Could you check a few things on this model? Use its own coordinates, in mm. A direction names the side the tool comes from. Give positions to 0.01 mm unless a question says otherwise; leave off trailing zeros. Order: outer loops, then holes, each group sorted by start corner. A loop starts at its lowest first (then second) coordinate and runs counter-clockwise, first axis right, second up. Notation, with made-up numbers: (18, 28) -> (61, 28) arc R16 cw to (61, 33) -> close; hole circle Ø1 at (38, -30). An arc over 180 degrees is marked (long way). One line per item, written item: value.
```python
from build123d import *

# Parameters (mm, degrees)
SKETCH1_R           = 1.75
BOSS_EXTRUDE1_DEPTH = 2


with BuildPart() as part:
    # Sketch1 → Boss-Extrude1 (new body)
    with BuildSketch(Plane(origin=(0, 0, 0), x_dir=(1, 0, 0), z_dir=(0, 1, 0))):
        with BuildLine():
            Line((-12.5, -149.799866489), (-12.5, -72.328332691))
            ThreePointArc((-12.5, -72.328332691), (-11.914213562, -70.914119129), (-10.5, -70.328332691))
            Line((-10.5, -70.328332691), (10.5, -70.328332691))
            ThreePointArc((10.5, -70.328332691), (11.914213562, -70.914119129), (12.5, -72.328332691))
            Line((12.5, -72.328332691), (12.5, -149.799866489))
            ThreePointArc((12.5, -149.799866489), (13.155638081, -151.280640283), (14.69269103, -151.790562389))
            ThreePointArc((14.69269103, -151.790562389), (132.068874077, -76.25), (138.800828598, 63.171037513))
            ThreePointArc((138.800828598, 63.171037513), (137.590696626, 64.247203361), (135.980489863, 64.074615697))
            Line((135.980489863, 64.074615697), (68.888173524, 25.338848798))
            ThreePointArc((68.888173524, 25.338848798), (67.370535433, 25.139047953), (66.156122716, 26.070899606))
            Line((66.156122716, 26.070899606), (55.656122716, 44.257433085))
            ThreePointArc((55.656122716, 44.257433085), (55.456321871, 45.775071175), (56.388173524, 46.989483893))
            Line((56.388173524, 46.989483893), (123.480489863, 85.725250792))
            ThreePointArc((123.480489863, 85.725250792), (124.435058545, 87.033436922), (124.108137568, 88.619524876))
            ThreePointArc((124.108137568, 88.619524876), (0, 152.5), (-124.108137568, 88.619524876))
            ThreePointArc((-124.108137568, 88.619524876), (-124.435058545, 87.033436922), (-123.480489863, 85.725250792))
            Line((-123.480489863, 85.725250792), (-56.388173524, 46.989483893))
            ThreePointArc((-56.388173524, 46.989483893), (-55.456321871, 45.775071175), (-55.656122716, 44.257433085))
            Line((-55.656122716, 44.257433085), (-66.156122716, 26.070899606))
            ThreePointArc((-66.156122716, 26.070899606), (-67.370535433, 25.139047953), (-68.888173524, 25.338848798))
            Line((-68.888173524, 25.338848798), (-135.980489863, 64.074615697))
            ThreePointArc((-135.980489863, 64.074615697), (-137.590696626, 64.247203361), (-138.800828598, 63.171037513))
            ThreePointArc((-138.800828598, 63.171037513), (-132.068874077, -76.25), (-14.69269103, -151.790562389))
            ThreePointArc((-14.69269103, -151.790562389), (-13.155638081, -151.280640283), (-12.5, -149.799866489))
        make_face()
        with Locations(Location((115.282765815, -66.558535876, 0), (0, 0, 270))):
            Circle(SKETCH1_R, mode=Mode.SUBTRACT)
        with Locations(Location((102.292384759, -59.058535876, 0), (0, 0, 270))):
            Circle(SKETCH1_R, mode=Mode.SUBTRACT)
        with Locations(Location((-115.282765815, -66.558535876, 0), (0, 0, 270))):
            Circle(SKETCH1_R, mode=Mode.SUBTRACT)
        with Locations(Location((-102.292384759, -59.058535876, 0), (0, 0, 270))):
            Circle(SKETCH1_R, mode=Mode.SUBTRACT)
        with Locations(Location((0, 133.117071753, 0), (0, 0, 270))):
            Circle(SKETCH1_R, mode=Mode.SUBTRACT)
        with Locations(Location((0, 118.117071753, 0), (0, 0, 270))):
            Circle(SKETCH1_R, mode=Mode.SUBTRACT)
        with Locations(Location((110.01987893, 90.400875942, 0), (0, 0, 270))):
            Circle(SKETCH1_R, mode=Mode.SUBTRACT)
        with Locations(Location((85.771167624, 76.400875942, 0), (0, 0, 270))):
            Circle(SKETCH1_R, mode=Mode.SUBTRACT)
        with Locations(Location((133.29987893, 50.078733142, 0), (0, 0, 270))):
            Circle(SKETCH1_R, mode=Mode.SUBTRACT)
        with Locations(Location((109.051167624, 36.078733142, 0), (0, 0, 270))):
            Circle(SKETCH1_R, mode=Mode.SUBTRACT)
        with Locations(Location((23.280000001, -140.480448046, 0), (0, 0, 270))):
            Circle(SKETCH1_R, mode=Mode.SUBTRACT)
        with Locations(Location((23.280000001, -112.480448046, 0), (0, 0, 270))):
            Circle(SKETCH1_R, mode=Mode.SUBTRACT)
        with Locations(Location((-23.279999999, -140.480448046, 0), (0, 0, 270))):
            Circle(SKETCH1_R, mode=Mode.SUBTRACT)
        with Locations(Location((-23.279999999, -112.480448046, 0), (0, 0, 270))):
            Circle(SKETCH1_R, mode=Mode.SUBTRACT)
        with Locations(Location((-133.299152367, 50.079152622, 0), (0, 0, 270))):
            Circle(SKETCH1_R, mode=Mode.SUBTRACT)
        with Locations(Location((-109.050441061, 36.079152622, 0), (0, 0, 270))):
            Circle(SKETCH1_R, mode=Mode.SUBTRACT)
        with Locations(Location((-110.019152367, 90.401295422, 0), (0, 0, 270))):
            Circle(SKETCH1_R, mode=Mode.SUBTRACT)
        with Locations(Location((-85.770441061, 76.401295422, 0), (0, 0, 270))):
            Circle(SKETCH1_R, mode=Mode.SUBTRACT)
        with BuildLine():
            Line((20.91, -89.999866489), (20.91, -39.999866489))
            ThreePointArc((20.91, -39.999866489), (22.66, -38.249866489), (24.41, -39.999866489))
            Line((24.41, -39.999866489), (24.41, -89.999866489))
            ThreePointArc((24.41, -89.999866489), (22.66, -91.749866489), (20.91, -89.999866489))
        make_face(mode=Mode.SUBTRACT)
        with BuildLine():
            Line((55.410000001, -89.999866489), (55.410000001, -39.999866489))
            ThreePointArc((55.410000001, -39.999866489), (53.660000001, -38.249866489), (51.910000001, -39.999866489))
            Line((51.910000001, -39.999866489), (51.910000001, -89.999866489))
            ThreePointArc((51.910000001, -89.999866489), (53.660000001, -91.749866489), (55.410000001, -89.999866489))
        make_face(mode=Mode.SUBTRACT)
        with BuildLine():
            Line((-105.647170717, -2.98653438), (-62.345900528, -27.98653438))
            ThreePointArc((-62.345900528, -27.98653438), (-59.955356071, -27.345989924), (-60.595900528, -24.955445467))
            Line((-60.595900528, -24.955445467), (-103.897170717, 0.044554533))
            ThreePointArc((-103.897170717, 0.044554533), (-106.287715174, -0.595989924), (-105.647170717, -2.98653438))
        make_face(mode=Mode.SUBTRACT)
        with BuildLine():
            Line((-90.147170716, 23.860253138), (-46.845900527, -1.139746862))
            ThreePointArc((-46.845900527, -1.139746862), (-44.45535607, -0.499202405), (-45.095900527, 1.891342051))
            Line((-45.095900527, 1.891342051), (-88.397170716, 26.891342051))
            ThreePointArc((-88.397170716, 26.891342051), (-90.787715173, 26.250797595), (-90.147170716, 23.860253138))
        make_face(mode=Mode.SUBTRACT)
        with BuildLine():
            Line((50.237170716, 92.986400869), (6.935900526, 67.986400869))
            ThreePointArc((6.935900526, 67.986400869), (6.29535607, 65.595856412), (8.685900526, 64.955311956))
            Line((8.685900526, 64.955311956), (51.987170716, 89.955311956))
            ThreePointArc((51.987170716, 89.955311956), (52.627715172, 92.345856412), (50.237170716, 92.986400869))
        make_face(mode=Mode.SUBTRACT)
        with BuildLine():
            Line((65.737170716, 66.139613351), (22.435900527, 41.139613351))
            ThreePointArc((22.435900527, 41.139613351), (21.79535607, 38.749068894), (24.185900527, 38.108524437))
            Line((24.185900527, 38.108524437), (67.487170716, 63.108524437))
            ThreePointArc((67.487170716, 63.108524437), (68.127715173, 65.499068894), (65.737170716, 66.139613351))
        make_face(mode=Mode.SUBTRACT)
    extrude(amount=BOSS_EXTRUDE1_DEPTH)


solid = part.part
```
1) Suppose I cut it at A-A, the plane z = -56.5. Write out the boundary of the cut face in (x, y), then the cut area to 3 significant figures.
Answer below:
outline: (-141.65, 0) -> (-122.86, 0) -> (-122.86, 2) -> (-141.65, 2) -> close; (-72.86, 0) -> (49.04, 0) -> (49.04, 2) -> (-72.86, 2) -> close; (56.04, 0) -> (72.86, 0) -> (72.86, 2) -> (56.04, 2) -> close; (122.86, 0) -> (141.65, 0) -> (141.65, 2) -> (122.86, 2) -> close
area: 353 mm2
2) Suppose I cut it at D-D, the plane y = 0.35. State how many separate pieces and enclosed holes the cut face has, then the cut area to 3 significant figures.
Answer below:
separate pieces: 1
enclosed holes: 24
area: 65,600 mm2
3) Suppose I cut it at B-B, the plane x = 80.5. Write out the boundary of the cut face in (y, z).
Answer below:
outline: (0, -129.52) -> (2, -129.52) -> (2, -60.91) -> (0, -60.91) -> close; (0, -32.04) -> (2, -32.04) -> (2, 129.52) -> (0, 129.52) -> close
4) Suppose I cut it at C-C, the plane z = 15. Write out the boundary of the cut face in (x, y).
Answer below:
outline: (-151.76, 0) -> (-84.84, 0) -> (-84.84, 2) -> (-151.76, 2) -> close; (-77.84, 0) -> (151.76, 0) -> (151.76, 2) -> (-77.84, 2) -> close
5) For P1, Ø3, axis at x = -109.05, z = -36.08, coming from the -Y side (3 decimals); P2, Ø1, axis at y = 1, z = 65.5, coming from the +X side; P3, Ø0.6, axis at x = -5, y = 1.5, coming from the +Z side, each with a flat end and sliding along its axis, tell me the tip position at first contact or that it passes through.
Answer below:
P1: passes through
P2: stops at x = 137.95
P3: stops at z = 70.33
6) For faces 5 (the flat face through (102.904, 0.986, -44.978)), 6 (the cylindrical face through (2.03, 0.986, -152.486)), which set-ups out of +Z, -Z, +X, -X, +Y, -Y let a thin tool reach every point of the face, with its end or its side?
Answer below:
face 5: +Y, -Y
face 6: -Z, +Y, -Y
7) We'd pull the mould along Z, two halves only. Please class faces 1 (the flat face through (-2, 2, -2)), 2 (the flat face through (45.53, 0.99, -50.43)), 3 (the flat face through (-68.8, 0.986, -11.535)), 4 (the cylindrical face through (131.042, 0.986, 78.001)): +Z half, -Z half, draft (parallel to the pull), parting line (faces both ways), or undercut.
Answer below:
face 1: draft
face 2: undercut
face 3: undercut
face 4: parting line
8) If I drill on line 1 along X through (y, z) = (1.15, 89.5); line 2 along X through (y, z) = (1.95, -89.5); line 3 along Z through (x, y) = (85, 0.7), over which ranges is the centre line in solid material (lowest first)?
Answer below:
line 1: x = -123.47 to -12.5, 12.5 to 20.91, 24.41 to 51.91, 55.41 to 123.47
line 2: x = -123.47 to -111.52, -108.52 to 44.2, 51.2 to 108.52, 111.52 to 123.47
line 3: z = -126.61 to -77.97, -74.83 to -63.51, -34.64 to 126.61
